Verification items for the finished model (mm, model axes). A direction names the side the tool comes from. Round coordinates to 2 decimals unless told otherwise and drop trailing zeros. Write each loop counter-clockwise with the first axis right and the second up, starting at its lowest first coordinate (ties: lowest second). Pieces come first, ordered by that corner, then holes.
from build123d import *

# Parameters (mm, degrees)
F0_W      = 50
F0_H      = 30
F1_DEPTH  = 10
F2_W      = 5
F2_H      = 5
F3_DEPTH  = 5
F5_DEPTH  = 20
F6_W      = 20
F6_H      = 20
F7_DEPTH  = 20
F8_R      = 7.5
F9_DEPTH  = 5
F10_R     = 7.5
F11_DEPTH = 5


with BuildPart() as f1:
    # F0 (on Top) → F1 (new body)
    with BuildSketch(Plane.XY):
        Rectangle(F0_W, F0_H)
    extrude(amount=F1_DEPTH)

    # F2 (on face) → F3 (join)
    with BuildSketch(Plane(origin=(0, 0, 0), x_dir=(1, 0, 0), z_dir=(0, 0, -1))):
        Polygon((-25, 2.5), (-25, 0), (-25, -2.5), (-20, -2.5), (-20, 2.5), align=None)
        with Locations((-7.5, 0)):
            Rectangle(F2_W, F2_H)
    extrude(amount=F3_DEPTH)

    # F4 (on face) → F5 (join)
    with BuildSketch(Plane.XY.offset(10)):
        Polygon((-5, 10), (-25, 10), (-25, 0), (-25, -10), (-5, -10), align=None)
    extrude(amount=F5_DEPTH)

    # F6 (on face) → F7 (join)
    with BuildSketch(Plane(origin=(-25, 0, 0), x_dir=(0, -1, 0), z_dir=(-1, 0, 0))):
        with Locations((0, 20)):
            Rectangle(F6_W, F6_H)
    extrude(amount=F7_DEPTH)

    # F8 (on face) → F9 (join)
    with BuildSketch(Plane.XZ.offset(10)):
        with Locations((-5, 30)):
            Circle(F8_R)
    extrude(amount=F9_DEPTH)

    # F10 (on face) → F11 (join)
    with BuildSketch(Plane(origin=(0, 10, 0), x_dir=(-1, 0, 0), z_dir=(0, 1, 0))):
        with Locations((5, 30)):
            Circle(F10_R)
    extrude(amount=F11_DEPTH)


solid = f1.part
Q1. Sectioned sample at D-D (z = 27). Enter the section's corners in (x, y).
Recorded:
outline: (-45, -10) - (-11.87, -10) - (-11.87, -15) - (1.87, -15) - (1.87, -10) - (-5, -10) - (-5, 10) - (1.87, 10) - (1.87, 15) - (-11.87, 15) - (-11.87, 10) - (-45, 10) - close
Q2. Release check for a two-part mould opening along Y. For faces 4 (the flat face through (-8, 2.5, -2)), 5 (the flat face through (-5, 0, 20)), 6 (the flat face through (0, -15, 5)) record: released by +Y, released by -Y, zero draft, split by the parting line, or undercut.
Recorded:
face 4: released by +Y
face 5: undercut
face 6: released by -Y
Q3. Depth check by flat-ended pin: P1, Ø8, axis at y = 0, z = 21, coming from the +X side; P2, Ø4, axis at x = -28.5, y = 4.5, coming from the -Z side; P3, Ø1.5, axis at y = -0.5, z = -2.5, coming from the -X side; P4, Ø4, axis at x = 1, z = 21, coming from the -Y side. Enter the tip coordinate at first touch or a pass-through.
Recorded:
P1: stops at x = -5
P2: stops at z = 10
P3: stops at x = -25
P4: passes through
Q4. Sectioned sample at C-C (y = 12). Enter the section's corners in (x, z), plus the area to 3 significant figures.
Recorded:
outline: (-25, 0) - (25, 0) - (25, 10) - (-25, 10) - close; circle Ø15 at (-5, 30)
area: 677 mm2
Q5. Material ranges on line 1 along Z through (x, y) = (-5, -11); line 2 along Z through (x, y) = (-35, -5.5); line 3 along Y through (x, z) = (-26, 16.5), recorded low to high.
Recorded:
line 1: z = 0 to 10, 22.5 to 37.5
line 2: z = 10 to 30
line 3: y = -10 to 10
Q6. Sectioned sample at B-B (x = -21). Enter the section's corners in (y, z), plus the area to 3 significant figures.
Recorded:
outline: (-15, 0) - (-2.5, 0) - (-2.5, -5) - (2.5, -5) - (2.5, 0) - (15, 0) - (15, 10) - (10, 10) - (10, 30) - (-10, 30) - (-10, 10) - (-15, 10) - close
area: 725 mm2
Q7. Tool access check on faces 1 (the flat face through (-10, 0, -2)), 2 (the flat face through (-25, 10, 20)), 3 (the flat face through (-23, 2.5, -2)). Record the directions out of +Z, -Z, +X, -X, +Y, -Y that give a thin tool (end or side, any length) a straight path to the whole face; none if there is none.
Recorded:
face 1: -Z, +Y, -Y
face 2: -X, +Y
face 3: -Z, +X, -X, +Y
Q8. Sectioned sample at A-A (y = 6.5). Enter the section's corners in (x, z).
Recorded:
outline: (-45, 10) - (-25, 10) - (-25, 0) - (25, 0) - (25, 10) - (-5, 10) - (-5, 30) - (-45, 30) - close
